Design review of the part built by this model. Coordinates are the model's own, in mm. Face numbers are marked on the shaded views. Give positions to 0.01 mm unless a question says otherwise; leave off trailing zeros. Loops run counter-clockwise (first coordinate to the right, second up) from the corner with the lowest first, then second, coordinate; pieces in that order, holes last.
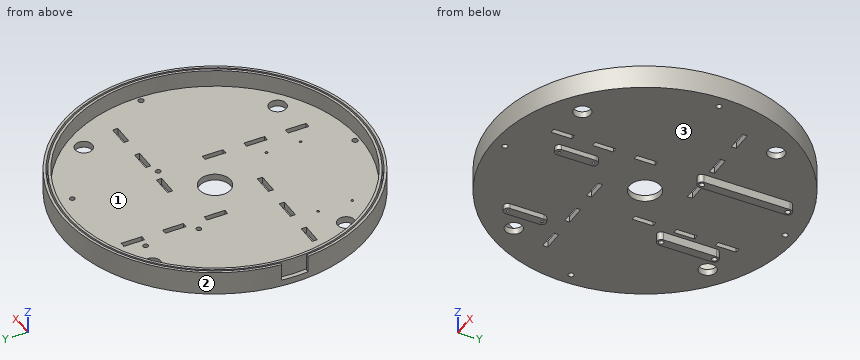
from build123d import *

# Parameters (mm, degrees)
SKETCH1_W                   = 200
SKETCH1_H                   = 200
SKETCH1_R                   = 9.15
BOSS_EXTRUDE1_DEPTH         = 3.75
SKETCH5_W                   = 12.1
SKETCH5_H                   = 3
SKETCH5_R                   = 5
CUT_EXTRUDE6_DEPTH          = 10
CIRPATTERN2_COUNT           = 4
SKETCH6_W                   = 200
SKETCH6_H                   = 200
SKETCH6_R                   = 88.610994186
CUT_EXTRUDE10_DEPTH         = 4.75
SKETCH7_R                   = 86.110994186
SKETCH7_R_2                 = 84.610994186
BOSS_EXTRUDE2_DEPTH         = 10
SKETCH11_R                  = 1.5
BOSS_EXTRUDE3_DEPTH         = 5
SKETCH13_R                  = 1.5
CUT_EXTRUDE11_DEPTH         = 14.75
SKETCH14_R                  = 0.75
BOSS_EXTRUDE4_DEPTH         = 3
SKETCH14_3_R                = 0.75
CUT_EXTRUDE12_DEPTH         = 14.75
TAP_DRILL_FOR_M4X0_7_TAP1_D = 3.3
CIRPATTERN3_COUNT           = 4


with BuildPart() as part:
    # Sketch1 → Boss-Extrude1 (new body)
    with BuildSketch(Plane.XY):
        Rectangle(SKETCH1_W, SKETCH1_H)
        Circle(SKETCH1_R, mode=Mode.SUBTRACT)
    extrude(amount=-BOSS_EXTRUDE1_DEPTH)

    # Sketch5 → Cut-Extrude6 (cut)
    with BuildSketch(Plane.XY):
        with Locations((35.9, 23.2)):
            Rectangle(SKETCH5_W, SKETCH5_H)
        with Locations((60.1, 23.2)):
            Rectangle(SKETCH5_W, SKETCH5_H)
        with Locations((11.7, 23.2)):
            Rectangle(SKETCH5_W, SKETCH5_H)
        with Locations((60.1, 44.7)):
            Circle(SKETCH5_R)
    cut_extrude6 = extrude(amount=-CUT_EXTRUDE6_DEPTH, mode=Mode.SUBTRACT)

    # CirPattern2: Cut-Extrude6 ×4 about axis
    cirpattern2_axis = Axis((0, 0, 0), (0, 0, 1))
    for i in range(1, CIRPATTERN2_COUNT):
        add(cut_extrude6.rotate(cirpattern2_axis, i * 360 / CIRPATTERN2_COUNT), mode=Mode.SUBTRACT)

    # Sketch6 → Cut-Extrude10 (cut, through all)
    with BuildSketch(Plane.XY):
        Rectangle(SKETCH6_W, SKETCH6_H)
        Circle(SKETCH6_R, mode=Mode.SUBTRACT)
    extrude(amount=-CUT_EXTRUDE10_DEPTH, mode=Mode.SUBTRACT)

    # Sketch7 → Boss-Extrude2 (add)
    with BuildSketch(Plane.XY):
        Circle(SKETCH7_R)
        Circle(SKETCH7_R_2, mode=Mode.SUBTRACT)
        with BuildLine():
            Line((-88.273802601, 7.722957014), (-86.779510554, 7.5922234))
            ThreePointArc((-86.779510554, 7.5922234), (87.110994186, 0), (-86.779510554, -7.5922234))
            Line((-86.779510554, -7.5922234), (-88.273802601, -7.722957014))
            ThreePointArc((-88.273802601, -7.722957014), (88.610994186, 0), (-88.273802601, 7.722957014))
        make_face()
    extrude(amount=BOSS_EXTRUDE2_DEPTH)

    # Sketch11 → Boss-Extrude3 (add)
    with BuildSketch(Plane(origin=(0, 0, -3.75), x_dir=(-1, 0, 0), z_dir=(0, 0, -1))):
        with BuildLine():
            Line((-26.4, 70.5), (-26.4, 20.5))
            ThreePointArc((-26.4, 20.5), (-23.9, 18), (-21.4, 20.5))
            Line((-21.4, 20.5), (-21.4, 70.5))
            ThreePointArc((-21.4, 70.5), (-23.9, 73), (-26.4, 70.5))
        make_face()
        with Locations((-23.9, 70.5)):
            Circle(SKETCH11_R, mode=Mode.SUBTRACT)
        with Locations((-23.9, 20.5)):
            Circle(SKETCH11_R, mode=Mode.SUBTRACT)
        with BuildLine():
            Line((27, 56), (27, 25))
            ThreePointArc((27, 25), (29.5, 22.5), (32, 25))
            Line((32, 25), (32, 56))
            ThreePointArc((32, 56), (29.5, 58.5), (27, 56))
        make_face()
        with Locations((29.5, 25)):
            Circle(SKETCH11_R, mode=Mode.SUBTRACT)
        with Locations((29.5, 56)):
            Circle(SKETCH11_R, mode=Mode.SUBTRACT)
    extrude(amount=BOSS_EXTRUDE3_DEPTH)

    # Sketch13 → Cut-Extrude11 (cut, through all)
    with BuildSketch(Plane(origin=(0, 0, -3.75), x_dir=(-1, 0, 0), z_dir=(0, 0, -1))):
        with Locations((29.5, 56)):
            Circle(SKETCH13_R)
        with Locations((29.5, 25)):
            Circle(SKETCH13_R)
        with Locations((-23.9, 20.5)):
            Circle(SKETCH13_R)
        with Locations((-23.9, 70.5)):
            Circle(SKETCH13_R)
    extrude(amount=-CUT_EXTRUDE11_DEPTH, mode=Mode.SUBTRACT)

    # Sketch14 → Boss-Extrude4 (add)
    with BuildSketch(Plane(origin=(0, 0, -3.75), x_dir=(-1, 0, 0), z_dir=(0, 0, -1))):
        with BuildLine():
            Line((-9.592467607, -36.349902261), (-9.592467607, -56.228581918))
            ThreePointArc((-9.592467607, -56.228581918), (-12.092467607, -58.728581918), (-14.592467607, -56.228581918))
            Line((-14.592467607, -56.228581918), (-14.592467607, -36.349902261))
            ThreePointArc((-14.592467607, -36.349902261), (-12.092467607, -33.849902261), (-9.592467607, -36.349902261))
        make_face()
        with Locations((-12.092467607, -56.228581918)):
            Circle(SKETCH14_R, mode=Mode.SUBTRACT)
        with Locations((-12.092467607, -36.349902261)):
            Circle(SKETCH14_R, mode=Mode.SUBTRACT)
        with BuildLine():
            Line((42.38621205, -36.349902261), (42.38621205, -56.228581918))
            ThreePointArc((42.38621205, -56.228581918), (44.88621205, -58.728581918), (47.38621205, -56.228581918))
            Line((47.38621205, -56.228581918), (47.38621205, -36.349902261))
            ThreePointArc((47.38621205, -36.349902261), (44.88621205, -33.849902261), (42.38621205, -36.349902261))
        make_face()
        with Locations((44.88621205, -36.349902261)):
            Circle(SKETCH14_R, mode=Mode.SUBTRACT)
        with Locations((44.88621205, -56.228581918)):
            Circle(SKETCH14_R, mode=Mode.SUBTRACT)
    extrude(amount=BOSS_EXTRUDE4_DEPTH)

    # Sketch14_3 → Cut-Extrude12 (cut, through all)
    with BuildSketch(Plane(origin=(0, 0, -3.75), x_dir=(-1, 0, 0), z_dir=(0, 0, -1))):
        with Locations((44.88621205, -36.349902261)):
            Circle(SKETCH14_3_R)
        with Locations((-12.092467607, -56.228581918)):
            Circle(SKETCH14_3_R)
        with Locations((-12.092467607, -36.349902261)):
            Circle(SKETCH14_3_R)
        with Locations((44.88621205, -56.228581918)):
            Circle(SKETCH14_3_R)
    extrude(amount=-CUT_EXTRUDE12_DEPTH, mode=Mode.SUBTRACT)

    # Tap Drill for M4x0.7 Tap1 (through all)
    with Locations(Plane.XY):
        with Locations((-81.610994186, 0)):
            tap_drill_for_m4x0_7_tap1 = Hole(TAP_DRILL_FOR_M4X0_7_TAP1_D / 2)

    # CirPattern3: Tap Drill for M4x0.7 Tap1 ×4 about axis
    cirpattern3_axis = Axis((0, 0, 0), (0, 0, 1))
    for i in range(1, CIRPATTERN3_COUNT):
        add(tap_drill_for_m4x0_7_tap1.rotate(cirpattern3_axis, i * 360 / CIRPATTERN3_COUNT), mode=Mode.SUBTRACT)


solid = part.part
Q1. Take a section at A-A (z = 3.75). Give the boundary of the cut face in (x, y).
Results:
outline: (-88.27, -7.72) arc R88.61 ccw (long way) to (-88.27, 7.72) - (-86.78, 7.59) arc R87.11 cw (long way) to (-86.78, -7.59) - close; circle Ø172.22 at (0, 0); hole circle Ø169.22 at (0, 0)
Q2. Wall thickness on line 1 (X direction, y = -60.1, z = -2.15); line 2 (X direction, y = 50.5, z = -6); line 3 (Y direction, x = 0, z = 3): over which ranges is each line inside the solid? List them lowest first.
Results:
line 1: x = -65.11 to 21.7, 24.7 to 39.7, 49.7 to 65.11
line 2: x = -32 to -27, 21.4 to 26.4
line 3: y = -88.61 to -87.11, -86.11 to -84.61, 84.61 to 86.11, 87.11 to 88.61
Q3. Take a section at B-B (y = 44.7). Give the boundary of the cut face in (x, z).
Results:
outline: (-76.51, -3.75) - (-32, -3.75) - (-32, -8.75) - (-27, -8.75) - (-27, -3.75) - (21.4, -3.75) - (21.4, -8.75) - (26.4, -8.75) - (26.4, -3.75) - (55.1, -3.75) - (55.1, 0) - (-71.84, 0) - (-71.84, 10) - (-73.6, 10) - (-73.6, 0) - (-74.77, 0) - (-74.77, 10) - (-76.51, 10) - close; (65.1, -3.75) - (76.51, -3.75) - (76.51, 10) - (74.77, 10) - (74.77, 0) - (73.6, 0) - (73.6, 10) - (71.84, 10) - (71.84, 0) - (65.1, 0) - close
Q4. Take a section at D-D (y = 14). Give the boundary of the cut face in (x, z), plus the area to 3 significant figures.
Results:
outline: (-87.5, -3.75) - (-24.7, -3.75) - (-24.7, 0) - (-83.44, 0) - (-83.44, 10) - (-84.97, 10) - (-84.97, 0) - (-85.98, 0) - (-85.98, 10) - (-87.5, 10) - close; (-21.7, -3.75) - (87.5, -3.75) - (87.5, 10) - (85.98, 10) - (85.98, 0) - (84.97, 0) - (84.97, 10) - (83.44, 10) - (83.44, 0) - (-21.7, 0) - close
area: 706 mm2
Q5. Draft analysis for pull direction Y (two halves, no side actions). For the marked faces 1, 2 and 3, state which applies: pulls with the +Y half, pulls with the -Y half, needs draft (parallel to the pull), parting line crosses it, or undercut.
Results:
face 1: undercut
face 2: parting line crosses it
face 3: needs draft
Q6. Take a section at C-C (x = -60.1). Give the boundary of the cut face in (y, z).
Results:
outline: (-65.11, -3.75) - (-49.7, -3.75) - (-49.7, 0) - (-59.56, 0) - (-59.56, 10) - (-61.67, 10) - (-61.67, 0) - (-63.06, 0) - (-63.06, 10) - (-65.11, 10) - close; (-39.7, -3.75) - (-24.7, -3.75) - (-24.7, 0) - (-39.7, 0) - close; (-21.7, -3.75) - (65.11, -3.75) - (65.11, 10) - (63.06, 10) - (63.06, 0) - (61.67, 0) - (61.67, 10) - (59.56, 10) - (59.56, 0) - (-21.7, 0) - close
Q7. Insertion check: pin 1 (4 mm diameter, centred on x = 61, z = -2.5, fed in from -Y); pin 2 (6 mm diameter, centred on x = 47, y = 7, fed in from +Z); pin 3 (1 mm diameter, centred on y = -48.5, z = 7.5, fed in from +X); pin 4 (1.2 mm diameter, centred on x = -44.89, y = -36.35, fed in from -Z). Each pin has a flat end and moves straight along its axis. Give the tip position at first contact, or say it passes through.
Results:
pin 1: stops at y = -66.11
pin 2: stops at z = 0
pin 3: stops at x = 74.48
pin 4: passes through
